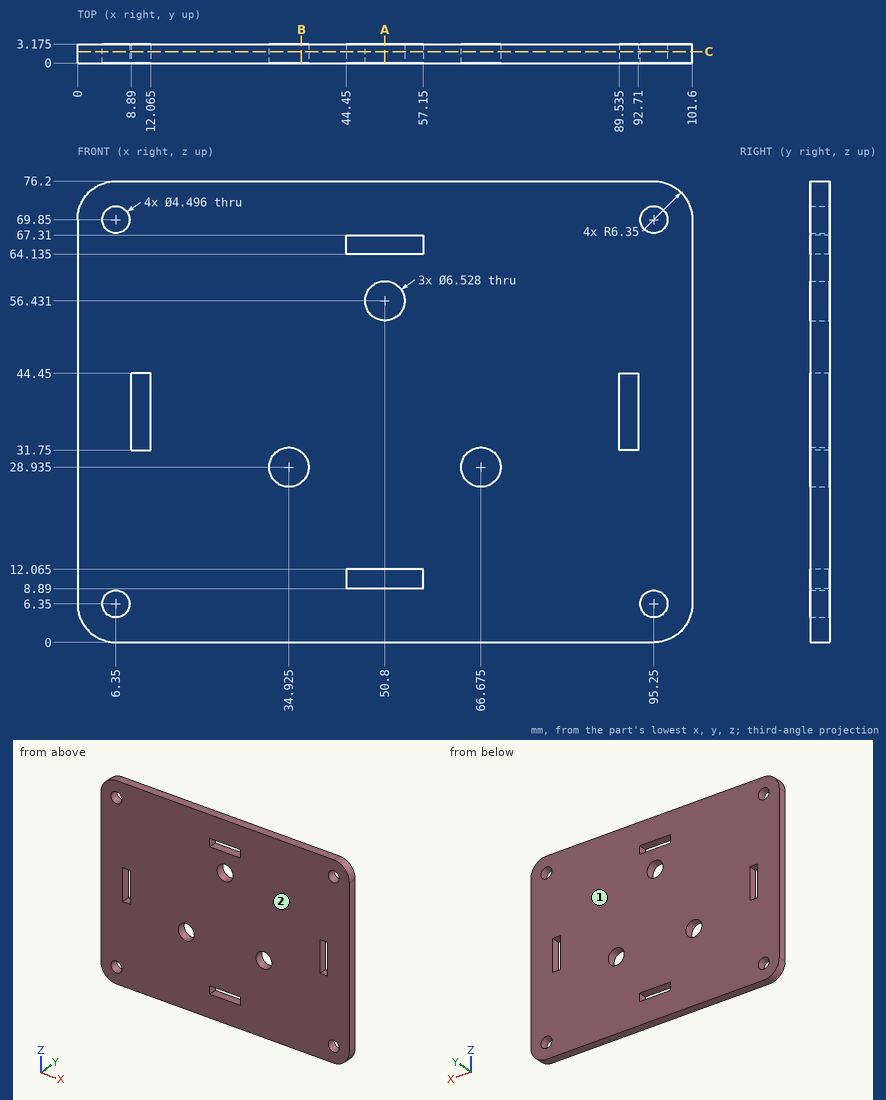
The figure shows three views and two pictorial views of one solid part (mm, origin at its lowest corner). Answer the questions. Give positions to 0.01 mm unless a question says otherwise; leave off trailing zeros. Order: outer loops, then holes, each group sorted by start corner. A loop starts at its lowest first (then second) coordinate and runs counter-clockwise, first axis right, second up. Notation, with made-up numbers: (23.25, -37) -> (34.25, -37) arc R29 cw to (34.25, -7) -> close; hole circle Ø5 at (37, 10.5). An arc over 180 degrees is marked (long way). Answer as CSV lines item,"result". Start each with the question number.
(1) For a pull along Y with two mould halves and no side action, classify the marked faces 1 and 2 as released by +Y, released by -Y, zero draft, split by the parting line, or undercut.
(2) Section B-B, the plane x = 37 is taken. Write down the section's boundary in (y, z) (1 decimal), plus the area to 3 significant figures.
(3) Consider line 1 along Z through (x, y) = (50.8, 2.35) (1 decimal); line 2 along X through (y, z) = (0.7, 66.5); line 3 along X through (y, z) = (2.25, 68.5). Determine where each line is inside the solid, lowest interval first.
(4) Section A-A, the plane x = 50.8 is taken. Write down the section's boundary in (y, z) (1 decimal), plus the area to 3 significant figures.
(5) Section C-C, the plane y = 1.9 is taken. Give the number of separate pieces and of enclosed holes in the cut face, plus the area to 3 significant figures.
Entries:
1,face 1,"released by +Y"
1,face 2,"released by -Y"
2,outline,"(0, 0) -> (3.2, 0) -> (3.2, 26.4) -> (0, 26.4) -> close; (0, 31.5) -> (3.2, 31.5) -> (3.2, 76.2) -> (0, 76.2) -> close"
2,area,"226 mm²"
3,line 1,"0 to 8.9, 12.1 to 53.2, 59.7 to 64.1, 67.3 to 76.2"
3,line 2,"0 to 44.45, 57.15 to 101.6"
3,line 3,"0 to 4.55, 8.15 to 93.45, 97.05 to 101.6"
4,outline,"(0, 0) -> (3.2, 0) -> (3.2, 8.9) -> (0, 8.9) -> close; (0, 12.1) -> (3.2, 12.1) -> (3.2, 53.2) -> (0, 53.2) -> close; (0, 59.7) -> (3.2, 59.7) -> (3.2, 64.1) -> (0, 64.1) -> close; (0, 67.3) -> (3.2, 67.3) -> (3.2, 76.2) -> (0, 76.2) -> close"
4,area,"201 mm²"
5,separate pieces,"1"
5,enclosed holes,"11"
5,area,"7,380 mm²"
